from build123d import *

# Parameters (mm, degrees)
SK_SHANK_R   = 1.25
SHANK_DEPTH  = 12
SK_HEAD_R    = 2.35
HEAD_DEPTH   = 1.3
HEAD_TAPER   = 26.84642782
SOCKET_START = 0.52
SOCKET_DEPTH = 1.28


with BuildPart() as part:
    # SK_shank → Shank (new body)
    with BuildSketch(Plane.XY):
        Circle(SK_SHANK_R)
    extrude(amount=-SHANK_DEPTH)

    # SK_head → Head (add)
    with BuildSketch(Plane.XY):
        Circle(SK_HEAD_R)
    extrude(amount=HEAD_DEPTH, taper=HEAD_TAPER)

    # SK_socket → Socket (cut)
    with BuildSketch(Plane.XY.offset(SOCKET_START)):
        Polygon((0.860251901, 0), (0.430125951, -0.745), (-0.430125951, -0.745), (-0.860251901, 0), (-0.430125951, 0.745), (0.430125951, 0.745), align=None)
    extrude(amount=SOCKET_DEPTH, mode=Mode.SUBTRACT)


solid = part.part
Can you work these out from the model? Positions are in its coordinate system, mm. Coordinates: 2 decimals unless noted, no trailing zeros. Write each loop counter-clockwise with the first axis right and the second up, starting at its lowest first coordinate (ties: lowest second). Pieces come first, ordered by that corner, then holes. Notation, with made-up numbers: (22, 44.25) -> (40, 44.25) arc R12 ccw to (40, 61.25) -> close; hole circle Ø10 at (87, -35.75). An arc over 180 degrees is marked (long way). Write each question's results on one line, items separated by ' | '. Start each with the question number.
Q1. I'm going to push flat-ended pins straight in: pin 1 (1 mm diameter, centred on x = 0, z = -1, fed in from +Y); pin 2 (1.5 mm diameter, centred on x = -0.5, z = 0, fed in from -Y); pin 3 (0.7 mm diameter, centred on x = 0, y = 0, fed in from +Z); pin 4 (2 mm diameter, centred on x = 1, z = -7.5, fed in from -Y). Where does each tip first touch, or does it pass through?
Q2. Imagine slicing it at A-A (x = 0). Write out the boundary of the cut face in (y, z) (3 decimals), then the cut area to 3 significant figures.
Q3. If I drill on probe 1 along Z at (x, y) = (0.3, -0.05); probe 2 along Y at (x, z) = (0.05, -8); probe 3 along Z at (x, y) = (-1.4, 0.1), over which ranges is the centre line in solid material (lowest first)?
Q4. Imagine slicing it at B-B (z = -10.5). Write out the boundary of the cut face in (x, y), then the cut area to 3 significant figures.
Q5. We'd pull the mould along Y, two halves only. Please class faces 1 (the face through (0, 0, 0.52)), 2 (the face through (-0.27, -1.22, -5.92)), 3 (the face through (1, -1, 0)): +Y half, -Y half, draft (parallel to the pull), parting line (faces both ways), or undercut.
Taken from the geometry:
1) pin 1: stops at y = 1.25 | pin 2: stops at y = -2.35 | pin 3: stops at z = 0.52 | pin 4: stops at y = -1.25
2) outline: (-2.35, 0) -> (-1.25, 0) -> (-1.25, -12) -> (1.25, -12) -> (1.25, 0) -> (2.35, 0) -> (1.692, 1.3) -> (0.745, 1.3) -> (0.745, 0.52) -> (-0.745, 0.52) -> (-0.745, 1.3) -> (-1.692, 1.3) -> close | area: 34.1 mm^2
3) probe 1: z = -12 to 0.52 | probe 2: y = -1.25 to 1.25 | probe 3: z = 0 to 1.3
4) outline: circle Ø2.5 at (0, 0) | area: 4.91 mm^2
5) face 1: undercut | face 2: parting line | face 3: draft
